```python
from build123d import *

# Parameters (mm, degrees)
BOSS_EXTRUDE1_DEPTH = 3
FILLET1_R           = 2
FILLET2_R           = 10
SKETCH2_W           = 3
SKETCH2_H           = 25
CUT_EXTRUDE1_DEPTH  = 10
SKETCH3_R           = 1
BOSS_EXTRUDE2_DEPTH = 3


with BuildPart() as part:
    # Sketch1 → Boss-Extrude1 (new body)
    with BuildSketch(Plane(origin=(0, 0, 0), x_dir=(1, 0, 0), z_dir=(0, 1, 0))):
        Polygon((0, 71.865), (0, -71.865), (292, -62.13), (292, 62.13), align=None)
        Polygon((15, 56.356580511), (60, 54.856323662), (60, -54.856323662), (15, -56.356580511), align=None, mode=Mode.SUBTRACT)
        Polygon((277, 47.621751744), (277, -47.621751744), (232, -49.122008593), (232, 49.122008593), align=None, mode=Mode.SUBTRACT)
        Polygon((75, 54.356238045), (75, -54.356238045), (217, -49.62209421), (217, 49.62209421), align=None, mode=Mode.SUBTRACT)
    extrude(amount=BOSS_EXTRUDE1_DEPTH)

    # Fillet1
    fillet1_edges = [part.edges().sort_by_distance(p)[0] for p in [
        (0, 1.5, 71.865),
        (0, 1.5, -71.865),
        (292, 1.5, -62.13),
        (292, 1.5, 62.13),
    ]]
    fillet(fillet1_edges, radius=FILLET1_R)

    # Fillet2
    fillet2_edges = [part.edges().sort_by_distance(p)[0] for p in [
        (217, 1.5, -49.62209421),
        (75, 1.5, -54.356238045),
        (75, 1.5, 54.356238045),
        (217, 1.5, 49.62209421),
        (15, 1.5, -56.356580511),
        (15, 1.5, 56.356580511),
        (60, 1.5, 54.856323662),
        (60, 1.5, -54.856323662),
        (277, 1.5, -47.621751744),
        (232, 1.5, -49.122008593),
        (232, 1.5, 49.122008593),
        (277, 1.5, 47.621751744),
    ]]
    fillet(fillet2_edges, radius=FILLET2_R)

    # Sketch2 → Cut-Extrude1 (cut)
    with BuildSketch(Plane(origin=(0, 3, 0), x_dir=(1, 0, 0), z_dir=(0, 1, 0))):
        Polygon((47.5, 70.281395548), (22.5, 71.114871575), (22.5, 68.114871575), (47.5, 67.281395548), align=None)
        Polygon((269.5, 62.880128425), (244.5, 63.713604452), (244.5, 60.713604452), (269.5, 59.880128425), align=None)
        with Locations((67.5, 37.5)):
            Rectangle(SKETCH2_W, SKETCH2_H)
        with Locations((224.5, 37.5)):
            Rectangle(SKETCH2_W, SKETCH2_H)
    cut_extrude1 = extrude(amount=-CUT_EXTRUDE1_DEPTH, mode=Mode.SUBTRACT)

    # Mirror1: Cut-Extrude1 across plane
    add(cut_extrude1.mirror(Plane.XY), mode=Mode.SUBTRACT)

    # Sketch3 → Boss-Extrude2 (add)
    with BuildSketch(Plane(origin=(0, 3, 0), x_dir=(1, 0, 0), z_dir=(0, 1, 0))):
        Polygon((38, 55.589782566), (60, 33.589782566), (61.509816897, 56.691838505), align=None)
        with Locations(Location((54, 49.589782566, 0), (0, 0, 270))):
            Circle(SKETCH3_R, mode=Mode.SUBTRACT)
        Polygon((232, 26.388549689), (254, 48.388549689), (229.701692371, 51.044206748), align=None)
        with Locations(Location((238, 42.388549689, 0), (0, 0, 270))):
            Circle(SKETCH3_R, mode=Mode.SUBTRACT)
        Polygon((254, -48.388549689), (229.701692371, -51.044206748), (232, -26.388549689), align=None)
        with Locations(Location((238, -42.388549689, 0), (0, 0, 90))):
            Circle(SKETCH3_R, mode=Mode.SUBTRACT)
        Polygon((60, -33.589782566), (61.509816897, -56.691838505), (38, -55.589782566), align=None)
        with Locations(Location((54, -49.589782566, 0), (0, 0, 90))):
            Circle(SKETCH3_R, mode=Mode.SUBTRACT)
    extrude(amount=-BOSS_EXTRUDE2_DEPTH)


solid = part.part
```
Build history of the part. All positions in model axes, mm. A direction names the side the tool comes from. Give positions to 0.01 mm unless a question says otherwise; leave off trailing zeros. Order: outer loops, then holes, each group sorted by start corner. A loop starts at its lowest first (then second) coordinate and runs counter-clockwise, first axis right, second up. Notation, with made-up numbers: M 34,11 L 71,11 A29 cw 71,47 Z; hole C 69,-21 d4. An arc over 180 degrees is marked long. Write item = value, one per line. Start each with the question number.
(1) Slice it at A-A on z = 9. Write the cut outline in (x, y).
(2) Which spindle directions (+Z, -Z, +X, -X, +Y, -Y) get a long thin tool onto all of the face, cutting with end or side? Do faces 1 (the flat face through (145, 0, 58)), 2 (the cylindrical face through (17.97, 1.52, 53.13)). Say none if no direction does.
(3) Slice it at D-D on z = -30.5. Write the cut outline in (x, y).
(4) Probe L1, parallel to X at y = 2.6, z = 10; L2, parallel to Z at x = 238, y = 0.8; L3, parallel to Z at x = 189, y = 0.85. List the from-to ranges inside material, lowest first. Write a range as [from, to].
(5) Two-plate mould, pull along X, no slides. Class faces 3 (the cylindrical face through (214.11, 1.52, 46.98)), 4 (the flat face through (145, 3, 58)): released by +X, released by -X, zero draft, split by the parting line, or undercut.
(6) Slice it at B-B on x = 182. Write the cut outline in (y, z).
(7) Slice it at C-C on y = 0.75. State how many separate pieces and enclosed holes the cut face has, plus the area to 3 significant figures.
(8) Pin check, flat tips, straight feed: pin 1 Ø1 at (x, y) = (65.5, 1) entering from +Z; pin 2 Ø1.2 at (x, z) = (54, -49.59) entering from +Y; pin 3 Ø0.9 at (x, y) = (224.5, 1.5) entering from +Z. Stop position of each tip, or through.
Responses:
q1.outline = M 0,0 L 15,0 L 15,3 L 0,3 Z; M 60,0 L 75,0 L 75,3 L 60,3 Z; M 217,0 L 232,0 L 232,3 L 217,3 Z; M 277,0 L 292,0 L 292,3 L 277,3 Z
q2.face_1 = +Z, -Z, +X, -X, -Y
q2.face_2 = +Y, -Y
q3.outline = M 0,0 L 15,0 L 15,3 L 0,3 Z; M 60,0 L 66,0 L 66,3 L 60,3 Z; M 69,0 L 75,0 L 75,3 L 69,3 Z; M 217,0 L 223,0 L 223,3 L 217,3 Z; M 226,0 L 236.11,0 L 236.11,3 L 226,3 Z; M 277,0 L 292,0 L 292,3 L 277,3 Z
q4.L1 = [0, 15], [60, 75], [217, 232], [277, 292]
q4.L2 = [-63.93, -43.39], [-41.39, -32.39], [32.39, 41.39], [43.39, 63.93]
q4.L3 = [-65.56, -50.56], [50.56, 65.56]
q5.face_3 = undercut
q5.face_4 = zero draft
q6.outline = M 0,-65.8 L 3,-65.8 L 3,-50.79 L 0,-50.79 Z; M 0,50.79 L 3,50.79 L 3,65.8 L 0,65.8 Z
q7.separate_pieces = 1
q7.enclosed_holes = 11
q7.area = 15,500 mm2
q8.pin_1 = 69.7
q8.pin_2 = through
q8.pin_3 = 64.4
